Model file for the job. Use its own axes, mm. Face numbers are marked on the shaded views. Round coordinates to 2 decimals unless told otherwise and drop trailing zeros. Write each loop counter-clockwise with the first axis right and the second up, starting at its lowest first coordinate (ties: lowest second). Pieces come first, ordered by that corner, then holes. Notation, with made-up numbers: (-9, -18.75) - (14, -18.75) arc R19 ccw to (14, 6.25) - close; hole circle Ø10 at (-12, 32.5). An arc over 180 degrees is marked (long way). Answer as a JSON object with one key per item and string values. Group by question number.
from build123d import *

# Parameters (mm, degrees)
SZKIC1_R                    = 2.5
DODANIE_WYCI_GNI_CIE1_DEPTH = 23.5
SFAZOWANIE1_SIZE            = 0.5
WYTNIJ_WYCI_GNI_CIE1_START  = -1.7
SZKIC2_R                    = 2.5
SZKIC2_R_2                  = 2.35
WYTNIJ_WYCI_GNI_CIE1_DEPTH  = 0.7
WYTNIJ_WYCI_GNI_CIE2_START  = -1
SZKIC3_R                    = 2.5
SZKIC3_R_2                  = 2.35
WYTNIJ_WYCI_GNI_CIE2_DEPTH  = 0.7


with BuildPart() as part:
    # Szkic1 → Dodanie-wyciągnięcie1 (new body)
    with BuildSketch(Plane.XY):
        Circle(SZKIC1_R)
    extrude(amount=DODANIE_WYCI_GNI_CIE1_DEPTH)

    # Sfazowanie1
    sfazowanie1_edges = [part.edges().sort_by_distance(p)[0] for p in [
        (-2.5, 0, 0),
        (-2.5, 0, 23.5),
    ]]
    chamfer(sfazowanie1_edges, length=SFAZOWANIE1_SIZE)

    # Szkic2 → Wytnij-wyciągnięcie1 (cut)
    with BuildSketch(Plane.XY.offset(23.5).offset(WYTNIJ_WYCI_GNI_CIE1_START)):
        Circle(SZKIC2_R)
        Circle(SZKIC2_R_2, mode=Mode.SUBTRACT)
    extrude(amount=WYTNIJ_WYCI_GNI_CIE1_DEPTH, mode=Mode.SUBTRACT)

    # Szkic3 → Wytnij-wyciągnięcie2 (cut)
    with BuildSketch(Plane(origin=(0, 0, 0), x_dir=(-1, 0, 0), z_dir=(0, 0, -1)).offset(WYTNIJ_WYCI_GNI_CIE2_START)):
        Circle(SZKIC3_R)
        with Locations(Location((0, 0, 0), (0, 0, 180))):
            Circle(SZKIC3_R_2, mode=Mode.SUBTRACT)
    extrude(amount=-WYTNIJ_WYCI_GNI_CIE2_DEPTH, mode=Mode.SUBTRACT)


solid = part.part
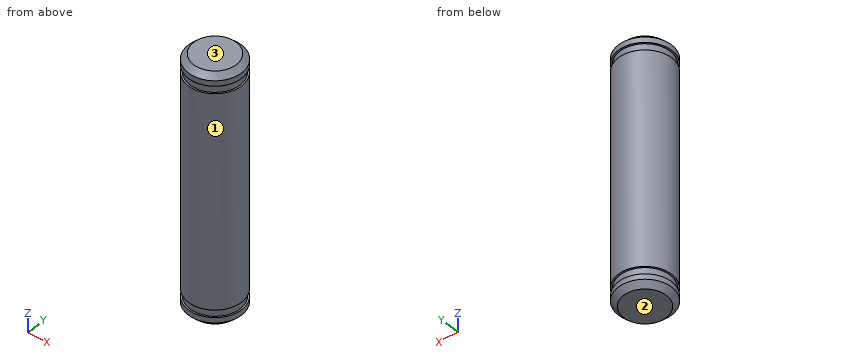
(1) Pull direction Z, two halves, no side cores. Call the marked faces 1, 2 and 3: pulls with the +Z half, pulls with the -Z half, needs draft (parallel to the pull), parting line crosses it, or undercut.
(2) Drill centre lines: line 1 (Z direction, x = -1.7, y = -1.7); line 2 (Y direction, x = 0.85, z = 4.75); line 3 (X direction, y = 0.2, z = 17). Where is each one in solid material? Low to high. Write a range as from..to.
(3) Flat gauge pins, fed straight in: pin 1 (3 mm diameter, centred on y = 2, z = 9.5, fed in from +X); pin 2 (2 mm diameter, centred on y = 0.5, z = 8, fed in from +X). Where does each tip first touch, or does it go through?
(4) Slice it at A-A (z = 7.25). Write the cut outline in (x, y).
Answer:
{
 "1": {"face 1": "needs draft", "face 2": "pulls with the -Z half", "face 3": "pulls with the +Z half"},
 "2": {"line 1": "0.4..1, 1.7..21.8, 22.5..23.1", "line 2": "-2.35..2.35", "line 3": "-2.49..2.49"},
 "3": {"pin 1": "x = 2.45", "pin 2": "x = 2.5"},
 "4": {"outline": "circle Ø5 at (0, 0)"}
}
